Work out the finished part from the listing and answer in its coordinate system (mm). Round coordinates to 2 decimals unless told otherwise and drop trailing zeros. Write each loop counter-clockwise with the first axis right and the second up, starting at its lowest first coordinate (ties: lowest second). Pieces come first, ordered by that corner, then holes. Notation, with made-up numbers: M -3,15.5 L 51,15.5 A17 ccw 51,20.5 Z; hole C -38.75,-7.75 d10. An arc over 180 degrees is marked long. Answer in a Markdown table with one row per item.
Autodesk Inventor part; units mm, degrees
ref_plane "YZ Plane" through (0, 0, 0) normal (1, 0, 0) x (0, 1, 0)
ref_plane "XZ Plane" through (0, 0, 0) normal (0, 1, 0) x (-1, 0, 0)
ref_plane "XY Plane" through (0, 0, 0) normal (0, 0, 1) x (1, 0, 0)
sketch "Sketch1" plane through (0, 0, 0) normal (0, 1, 0) x (-1, 0, 0)
  circle A0 centre (0, 0) radius 165.1
  circle A1 centre (0, 0) radius 129.54
  dimension "d0" = 330.2
  dimension "d1" = 259.08
extrude "Extrusion1" add sketch "Sketch1" along normal blind 12.7
sketch "Sketch2" plane through (0, 12.7, 0) normal (0, 1, 0) x (1, 0, 0)
  circle A0 centre (19.05, -152.4) radius 4.7802
  line L0 (0, 0) -> (0, -55.3703) construction
  circle A1 centre (-19.05, -152.4) radius 4.7802
  dimension "d6" = 152.4
  dimension "d7" = 19.05
hole "Hole1" at (19.05, 12.7, 152.4) at (-19.05, 12.7, 152.4) direction (0, -1, 0) diameter 5.3594 end through all
pattern_circular "Circular Pattern1" count 4 over 360 about axis through (0, -10, 0) along (0, 1, 0) of "Hole1"
sketch "Sketch3" plane through (0, 12.7, 0) normal (0, 1, 0) x (1, 0, 0)
  line L0 (0, 0) -> (103.2729, 103.2729) construction
  line L1 (0, 0) -> (146.05, 0) construction
  circle A0 centre (103.2729, 103.2729) radius 4.2786
  dimension "d18" = 146.05
  dimension "d19" = 45
hole "Hole2" at (103.2729, 12.7, -103.2729) direction (0, -1, 0) diameter 8.4328 end through all
pattern_circular "Circular Pattern2" count 4 over 360 about axis through (0, 0, 0) along (0, 1, 0) of "Hole2"
properties part number "fixedRing"
1. Consider line 1 along Z through (x, y) = (-18, 6.5); line 2 along Z through (x, y) = (-152.4, 4.5). Determine where each line is inside the solid, lowest interval first. Write a range as from..to.
Calculated:
| item | result |
|---|---|
| line 1 | z = -164.12..-154.87, -149.93..-128.28, 128.28..149.93, 154.87..164.12 |
| line 2 | z = -63.5..-21.73, -16.37..16.37, 21.73..63.5 |
2. Determine the mould class of faces 1 (the flat face through (99, 0, -85)), 2 (the cylindrical face through (106.38, 6.26, 100.42)), 3 (the cylindrical face through (35.79, 6.261, 161.174)) for opening direction X: released by +X, released by -X, zero draft, split by the parting line, or undercut.
Calculated:
| item | result |
|---|---|
| face 1 | zero draft |
| face 2 | undercut |
| face 3 | split by the parting line |
3. The part is cut by section C-C (y = 5.5). Count the separate pieces of the cut face and the enclosed holes in it, plus the area to 3 significant figures.
Calculated:
| item | result |
|---|---|
| separate pieces | 1 |
| enclosed holes | 13 |
| area | 32,500 mm² |
4. Given pin 1 (5 mm diameter, centred on x = -102, y = 7.5, fed in from -Z); pin 2 (1.5 mm diameter, centred on y = 11, z = 43, fed in from +X); pin 3 (4.5 mm diameter, centred on x = -152.4, z = 19.05, fed in from -Y); pin 4 (2 mm diameter, centred on y = 8, z = 105.5, fed in from -X), each flat-ended and moving along its own axis, determine where each tip first touches the part or whether it passes through.
Calculated:
| item | result |
|---|---|
| pin 1 | stops at z = -131.75 |
| pin 2 | stops at x = 159.6 |
| pin 3 | passes through |
| pin 4 | stops at x = -127.82 |
5. The part is cut by section A-A (x = 0). Determine the outline of the cut face in (y, z), plus the area to 3 significant figures.
Calculated:
| item | result |
|---|---|
| outline | M 0,-165.1 L 12.7,-165.1 L 12.7,-129.54 L 0,-129.54 Z; M 0,129.54 L 12.7,129.54 L 12.7,165.1 L 0,165.1 Z |
| area | 903 mm² |
6. The part is cut by section B-B (z = -75). Determine the outline of the cut face in (x, y).
Calculated:
| item | result |
|---|---|
| outline | M -147.08,0 L -105.62,0 L -105.62,12.7 L -147.08,12.7 Z; M 105.62,0 L 147.08,0 L 147.08,12.7 L 105.62,12.7 Z |
